Autodesk Inventor part; units mm, degrees
ref_plane "Start plane" through (0, 0, 85) normal (0, 0, 1) x (1, 0, 0)
ref_plane "End plane" through (0, 0, 1555) normal (0, 0, 1) x (1, 0, 0)
ref_plane "Work Plane4" through (-55, 0, 1555) normal (0.7071, 0, 0.7071) x (0.7071, 0, -0.7071)
ref_plane "Start plane" through (0, 0, 85) normal (0, 0, 1) x (1, 0, 0)
ref_plane "End plane" through (0, 0, 1555) normal (0, 0, 1) x (1, 0, 0)
sketch "Sketch2" plane through (0, 0, 0) normal (0, 0, 1) x (1, 0, 0)
  line L0 (-55, 100.8) -> (-14.95, 100.8)
  line L1 (-55, 110) -> (-55, 100.8)
  line L2 (55, 110) -> (-55, 110)
  line L3 (55, 100.8) -> (55, 110)
  line L4 (14.95, 100.8) -> (55, 100.8)
  line L5 (2.95, -88.8) -> (2.95, 88.8)
  line L6 (55, -100.8) -> (14.95, -100.8)
  line L7 (55, -110) -> (55, -100.8)
  line L8 (-55, -100.8) -> (-55, -110)
  line L9 (-14.95, -100.8) -> (-55, -100.8)
  line L10 (-2.95, 88.8) -> (-2.95, -88.8)
  line L11 (0, -154) -> (0, 154) construction
  line L12 (-2.95, -100.8) -> (2.95, -100.8) construction
  arc A0 (-14.95, -100.8) -> (-2.95, -88.8) centre (-14.95, -88.8) ccw
  arc A1 (-2.95, 88.8) -> (-14.95, 100.8) centre (-14.95, 88.8) ccw
  arc A2 (14.95, 100.8) -> (2.95, 88.8) centre (14.95, 88.8) ccw
  arc A3 (2.95, -88.8) -> (14.95, -100.8) centre (14.95, -88.8) ccw
  line L13 (-77, 0) -> (77, 0) construction
  line L14 (-55, -110) -> (55, -110)
  point P0 (-2.95, 100.8)
  point P1 (2.95, 100.8)
  point P2 (0, 0)
  point P3 (0, -100.8)
  point P4 (0, 0)
  dimension "d1" = 220
  dimension "d3" = 9.2
  dimension "d5" = 5.9
  dimension "d7" = 110
  dimension "d13" = 12
  dimension "d14" = 110
  dimension "d15" = 55
extrude "Body" add sketch "Sketch2" along normal up to surface (1470 mm away) from surface at 85
sketch "Sketch3" plane through (0, 0, 0) normal (0, 0, 1) x (1, 0, 0)
  line L0 (0, 0) -> (10, 0)
ref_plane "Work Plane3" through (0, 0, 0) normal (0, -1, 0) x (1, 0, 0)
ref_plane "Work Plane4" through (-55, 0, 1555) normal (0.7071, 0, 0.7071) x (0.7071, 0, -0.7071)
split "Split1" plane through (-55, 0, 1555) removes the side toward (0.7071, 0, 0.7071)
ref_plane "Work Plane5" through (0, 4000, 85) normal (0, 0, -1) x (-1, 0, 0)
split "Split2" plane through (0, 4000, 85) removes the side toward (0, 0, -1)
sketch "Sketch4" plane through (0, 0, 0) normal (0, -1, 0) x (1, 0, 0)
  line L0 (-2, 85) -> (12, 85)
  line L1 (-2, 1555) -> (12, 1555)
  dimension "d19" = 1470
equation "\"d1\" = ParH"
equation "\"d3\" = t2"
equation "\"d7\" = b"
equation "\"d13\" = R1"
equation "\"d14\" = 0.5 * d1"
equation "\"d15\" = 0.5 * d7"
equation "\"d8\" = G_L"
equation "\"b\" = 110"
equation "\"ParH\" = 220"
equation "\"R1\" = 12"
equation "\"G_L\" = d19"
equation "\"t1\" = 5.9"
equation "\"t2\" = 9.2"
equation "\"G_OFFSET_START\" = -85"
equation "\"G_OFFSET_END\" = 55"
equation "\"d16\" = -G_OFFSET_START"
equation "\"d17\" = G_OFFSET_END + B_L"
properties part number "DIN 1025 - IPE 220-1470" material "Steel, Mild"
The listing builds one solid part. Answer for the finished solid, in the listing's coordinates (mm). A direction names the side the tool comes from. Give positions to 0.01 mm unless a question says otherwise; leave off trailing zeros. Write each loop counter-clockwise with the first axis right and the second up, starting at its lowest first coordinate (ties: lowest second). Pieces come first, ordered by that corner, then holes.
1) Given P1, Ø12, axis at y = 7, z = 1361.5, coming from the -X side, flat-ended and moving along its own axis, determine where the tip first touches the part or whether it passes through.
2) Section B-B (z = 423.5) is taken. Write down the section's boundary in (x, y), and give its area (3 significant figures).
3) Section A-A (x = 30) is taken. Write down the section's boundary in (y, z).
4) Find the intervals of material crossed by L1, parallel to Y at x = 28.5, z = 906.5; L2, parallel to X at y = -65.5, z = 831.5; L3, parallel to Y at x = -4.5, z = 628.5, in increasing order.
5) Section C-C (y = -48) is taken. Write down the section's boundary in (x, z), and give its area (3 significant figures).
6) A tool of negligible diameter and unlimited length cuts with its end or side. For faces 5 (the face through (-35, 100.8, 810)), 6 (the face through (2.95, -1, 781)), 7 (the face through (0, -1, 1500)), from which of +Z, -Z, +X, -X, +Y, -Y can it reach the whole face along a straight path? Write none if from no direction.
7) For a pull along Y with two mould halves and no side action, classify faces 1 (the face through (0, 1, 85)), 2 (the face through (-35, -100.8, 810)), 3 (the face through (-1, -110, 810)), 4 (the face through (-2.95, 1, 784)) as pulls with the +Y half, pulls with the -Y half, needs draft (parallel to the pull), parting line crosses it, or undercut.
Response:
1. P1: stops at x = -2.95
2. outline: (-55, -110) - (55, -110) - (55, -100.8) - (14.95, -100.8) arc R12 cw to (2.95, -88.8) - (2.95, 88.8) arc R12 cw to (14.95, 100.8) - (55, 100.8) - (55, 110) - (-55, 110) - (-55, 100.8) - (-14.95, 100.8) arc R12 cw to (-2.95, 88.8) - (-2.95, -88.8) arc R12 cw to (-14.95, -100.8) - (-55, -100.8) - close
2. area: 3,340 mm2
3. outline: (-110, 85) - (-100.8, 85) - (-100.8, 1470) - (-110, 1470) - close; (100.8, 85) - (110, 85) - (110, 1470) - (100.8, 1470) - close
4. L1: y = -110 to -100.8, 100.8 to 110
4. L2: x = -2.95 to 2.95
4. L3: y = -110 to -94.7, 94.7 to 110
5. outline: (-2.95, 85) - (2.95, 85) - (2.95, 1497.05) - (-2.95, 1502.95) - close
5. area: 8,350 mm2
6. face 5: +Z, -Z, -X
6. face 6: +Z, -Z, +X
6. face 7: +Z, +X, +Y, -Y
7. face 1: needs draft
7. face 2: undercut
7. face 3: pulls with the -Y half
7. face 4: undercut
